Source: CAD feature listing. Evaluate the final solid. Frame: model axes, mm. A direction names the side the tool comes from. Round coordinates to 2 decimals unless told otherwise and drop trailing zeros. Loops run counter-clockwise (first coordinate to the right, second up) from the corner with the lowest first, then second, coordinate; pieces in that order, holes last. Notation, with made-up numbers: (18.5, -6.75) -> (77.5, -6.75) arc R9 cw to (77.5, 1.25) -> close; hole circle Ø1 at (58.25, -32.75). An arc over 180 degrees is marked (long way). Return JSON: item names as keys, results as strings. Group by question number.
```python
from build123d import *

# Parameters (mm, degrees)
BOSS_EXTRUDE1_DEPTH = 9.5
SKETCH1_3_R         = 2.75
BOSS_EXTRUDE2_DEPTH = 5
CUT_EXTRUDE2_DEPTH  = 16
SKETCH7_R           = 0.5
BOSS_EXTRUDE3_DEPTH = 0.5


with BuildPart() as part:
    # Sketch1 → Boss-Extrude1 (new body)
    with BuildSketch(Plane(origin=(0, 0, 0), x_dir=(1, 0, 0), z_dir=(0, 1, 0))):
        with BuildLine():
            Line((8.08, 7.5), (-8.08, 7.5))
            Line((-8.08, 7.5), (-8.08, 5.153988747))
            ThreePointArc((-8.08, 5.153988747), (-4.5, 0), (-8.08, -5.153988747))
            Line((-8.08, -5.153988747), (-8.08, -7.5))
            Line((-8.08, -7.5), (8.08, -7.5))
            Line((8.08, -7.5), (8.08, -5.153988747))
            ThreePointArc((8.08, -5.153988747), (4.5, 0), (8.08, 5.153988747))
            Line((8.08, 5.153988747), (8.08, 7.5))
        make_face()
    extrude(amount=BOSS_EXTRUDE1_DEPTH)

    # Sketch1_3 → Boss-Extrude2 (add)
    with BuildSketch(Plane(origin=(0, 0, 0), x_dir=(1, 0, 0), z_dir=(0, 1, 0))):
        with BuildLine():
            Line((-8.08, 5.153988747), (-8.08, 7.5))
            Line((-8.08, 7.5), (-10, 7.5))
            ThreePointArc((-10, 7.5), (-17.5, 0), (-10, -7.5))
            Line((-10, -7.5), (-8.08, -7.5))
            Line((-8.08, -7.5), (-8.08, -5.153988747))
            ThreePointArc((-8.08, -5.153988747), (-4.5, 0), (-8.08, 5.153988747))
        make_face()
        with Locations((-10, 0)):
            Circle(SKETCH1_3_R, mode=Mode.SUBTRACT)
        with BuildLine():
            Line((10, 7.5), (8.08, 7.5))
            Line((8.08, 7.5), (8.08, 5.153988747))
            ThreePointArc((8.08, 5.153988747), (4.5, 0), (8.08, -5.153988747))
            Line((8.08, -5.153988747), (8.08, -7.5))
            Line((8.08, -7.5), (10, -7.5))
            ThreePointArc((10, -7.5), (17.5, 0), (10, 7.5))
        make_face()
        with Locations((10, 0)):
            Circle(SKETCH1_3_R, mode=Mode.SUBTRACT)
    extrude(amount=BOSS_EXTRUDE2_DEPTH)

    # Sketch3 → Cut-Extrude2 (cut, through all)
    with BuildSketch(Plane.XY.offset(7.5)):
        with BuildLine():
            Line((1.6e-08, 9.5), (-8.08, 9.5))
            Line((-8.08, 9.5), (-8.08, 5))
            ThreePointArc((-8.08, 5), (-4.624294534, 8.299133313), (1.6e-08, 9.5))
        make_face()
        with BuildLine():
            Line((8.08, 9.5), (1.6e-08, 9.5))
            ThreePointArc((1.6e-08, 9.5), (4.624294548, 8.299133305), (8.08, 5))
            Line((8.08, 5), (8.08, 9.5))
        make_face()
        with BuildLine():
            Line((-4.1, 0), (4.1, 0))
            ThreePointArc((4.1, 0), (0, 4.1), (-4.1, 0))
        make_face()
        with BuildLine():
            ThreePointArc((-4.1, 0), (0, -4.1), (4.1, 0))
            Line((4.1, 0), (-4.1, 0))
        make_face()
    extrude(amount=-CUT_EXTRUDE2_DEPTH, mode=Mode.SUBTRACT)

    # Sketch7 → Boss-Extrude3 (add, symmetric)
    with BuildSketch(Plane.XY):
        with Locations((0, 9.5)):
            Circle(SKETCH7_R)
    extrude(amount=BOSS_EXTRUDE3_DEPTH, both=True)


solid = part.part
```
(1) Mould query, pull axis X, two halves, no side actions, for faces 1 (the face through (17.5, 2.46, 0.16)), 2 (the face through (12.54, 2.46, 1.05)), 3 (the face through (0, 5, 7.5)), 4 (the face through (-17.5, 2.46, -0.16)). Classes: released by +X, released by -X, zero draft, split by the parting line, or undercut.
(2) Cut plane C-C (x = 11.5). Return loops of the section in (y, z), and give its area (3 significant figures).
(3) Set-up query: faces 5 (the face through (-13, 5, -2)), 6 (the face through (12.4, 5, -1.8)), 7 (the face through (7.7, 0, -1.8)). Return all of +Z, -Z, +X, -X, +Y, -Y with unobstructed straight access to the full face (end or side cutting, diameter ignored); none if empty.
(4) Cut plane B-B (z = 1.5). Return loops of the section in (x, y), and give its area (3 significant figures).
(5) Pin query (flat end, axial travel): pin 1 (1.5 mm diameter, centred on y = 5.5, z = -3.5, fed in from +X); pin 2 (5 mm diameter, centred on x = -0.5, z = -3.5, fed in from -Y); pin 3 (2 mm diameter, centred on y = 2.5, z = 4.5, fed in from -X). Return the tip coordinate at first contact, or that it passes through.
(6) Cut plane D-D (y = 1). Return loops of the section in (x, z).
(7) Cut plane A-A (y = 3.75). Return loops of the section in (x, z), and give its area (3 significant figures).
(8) Ray query, line 1 (Z direction, x = 10, y = 2.6); line 2 (X direction, y = 1.9, z = 0); line 3 (X direction, y = 2.75, z = 0). Return the intervals inside material, ascending.
Answers follow:
{
 "1": {"face 1": "released by +X", "face 2": "undercut", "face 3": "zero draft", "face 4": "released by -X"},
 "2": {"outline": "(0, -7.35) -> (5, -7.35) -> (5, -2.3) -> (0, -2.3) -> close; (0, 2.3) -> (5, 2.3) -> (5, 7.35) -> (0, 7.35) -> close", "area": "50.4 mm^2"},
 "3": {"face 5": "-X, +Y", "face 6": "+X, +Y", "face 7": "+Z, -Z, +X, -X, -Y"},
 "4": {"outline": "(-17.35, 0) -> (-12.3, 0) -> (-12.3, 5) -> (-17.35, 5) -> close; (-7.7, 0) -> (-4.1, 0) arc R4.1 cw to (4.1, 0) -> (7.7, 0) -> (7.7, 5) -> (4.71, 5) -> (4.71, 8.25) arc R9.5 ccw to (-4.71, 8.25) -> (-4.71, 5) -> (-7.7, 5) -> close; (12.3, 0) -> (17.35, 0) -> (17.35, 5) -> (12.3, 5) -> close", "area": "140 mm^2"},
 "5": {"pin 1": "x = 16.9", "pin 2": "y = 2.79", "pin 3": "x = -16.63"},
 "6": {"outline": "(-10, -7.5) -> (-3.98, -7.5) -> (-3.98, 7.5) -> (-10, 7.5) arc R7.5 ccw to start; (3.98, -7.5) -> (10, -7.5) arc R7.5 ccw to (10, 7.5) -> (3.98, 7.5) -> close; hole circle Ø5.5 at (-10, 0); hole circle Ø5.5 at (10, 0)"},
 "7": {"outline": "(-10, -7.5) -> (-1.66, -7.5) -> (-1.66, 7.5) -> (-10, 7.5) arc R7.5 ccw to start; (1.66, -7.5) -> (10, -7.5) arc R7.5 ccw to (10, 7.5) -> (1.66, 7.5) -> close; hole circle Ø5.5 at (-10, 0); hole circle Ø5.5 at (10, 0)", "area": "379 mm^2"},
 "8": {"line 1": "-7.5 to -2.75, 2.75 to 7.5", "line 2": "-17.5 to -12.75, -7.25 to -3.63, 3.63 to 7.25, 12.75 to 17.5", "line 3": "-17.5 to -12.75, -7.25 to -3.04, 3.04 to 7.25, 12.75 to 17.5"}
}
